Can you work these out from the drawing? Everything is in mm from the part's minimum corner. A direction names the side the tool comes from. Give positions to 0.01 mm unless a question says otherwise; leave off trailing zeros. Write each loop counter-clockwise with the first axis right and the second up, starting at its lowest first coordinate (ties: lowest second). Pieces come first, ordered by that corner, then holes. Notation, with made-up numbers: M -20,25.5 L 8,25.5 A15 ccw 8,52.5 Z; hole C 87,32 d5. An arc over 180 degrees is marked long. One line per item, written item: value.
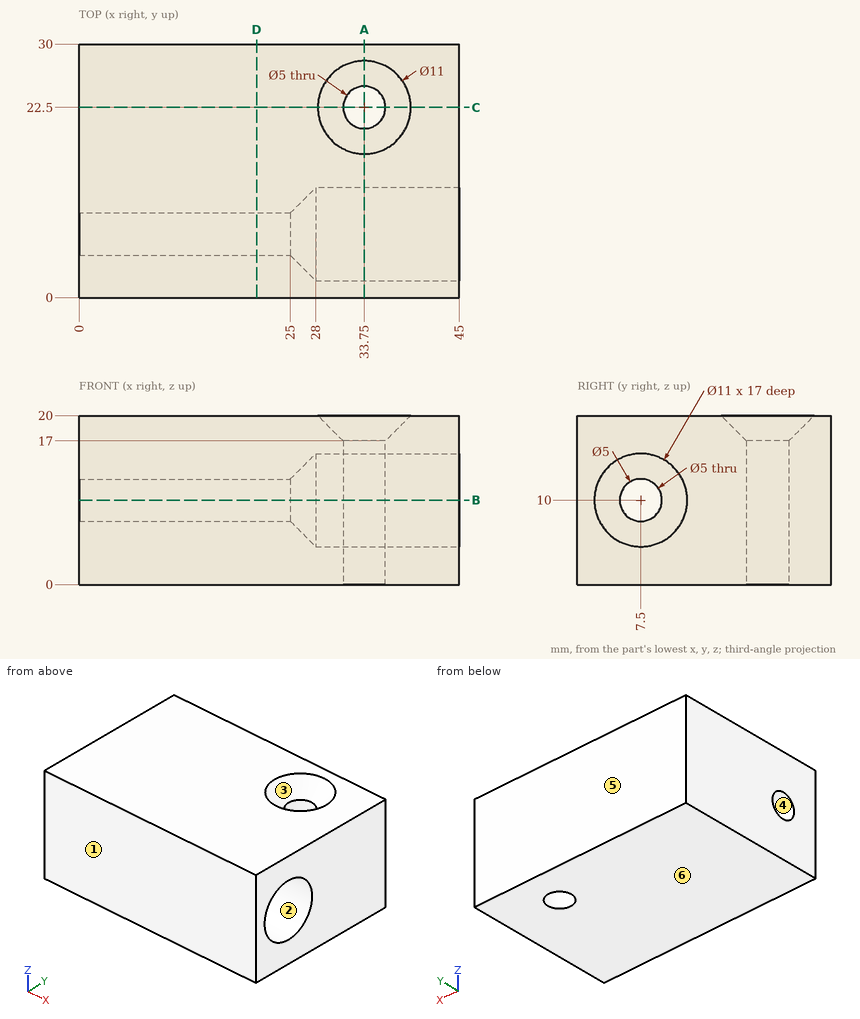
1) I'm going to push flat-ended pins straight in: pin 1 (2 mm diameter, centred on y = 7.5, z = 7.5, fed in from +X); pin 2 (9 mm diameter, centred on y = 7.5, z = 10, fed in from +X). Where does each tip first touch, or does it pass through?
Outcome:
pin 1: stops at x = 26
pin 2: stops at x = 27
2) We'd pull the mould along Y, two halves only. Please class the marked faces 3, 4, 5 and 6: pulls with the +Y half, pulls with the -Y half, needs draft (parallel to the pull), parting line crosses it, or undercut.
Outcome:
face 3: undercut
face 4: undercut
face 5: pulls with the +Y half
face 6: needs draft
3) Please list where these lines run through material, in increasing order: L1, parallel to Y at x = 33.75, z = 8.5; L2, parallel to Y at x = 33.75, z = 6.25; L3, parallel to Z at x = 8.25, y = 7.5. Write a range as from..to.
Outcome:
L1: y = 0..2.21, 12.79..20, 25..30
L2: y = 0..3.48, 11.52..20, 25..30
L3: z = 0..7.5, 12.5..20
4) If we section it at C-C, the plane y = 22.5: Write out the boundary of the cut face in (x, z).
Outcome:
outline: M 0,0 L 31.25,0 L 31.25,17 L 28.25,20 L 0,20 Z; M 36.25,0 L 45,0 L 45,20 L 39.25,20 L 36.25,17 Z
5) If we section it at D-D, the plane x = 21: Write out the boundary of the cut face in (y, z).
Outcome:
outline: M 0,0 L 30,0 L 30,20 L 0,20 Z; hole C 7.5,10 d5
6) If we section it at A-A, the plane x = 33.75: Write out the boundary of the cut face in (y, z).
Outcome:
outline: M 0,0 L 20,0 L 20,17 L 17,20 L 0,20 Z; M 25,0 L 30,0 L 30,20 L 28,20 L 25,17 Z; hole C 7.5,10 d11
7) On a 3-axis mill with a long thin cutter (end or side, diameter ignored), from which of +Z, -Z, +X, -X, +Y, -Y can I reach the whole of each face in a straight line? I mean the marked faces 1 and 2. Say none if no direction works.
Outcome:
face 1: +Z, -Z, +X, -X, -Y
face 2: +X
8) If we section it at B-B, the plane z = 10: Give the number of separate pieces and of enclosed holes in the cut face, then the cut area to 3 significant figures.
Outcome:
separate pieces: 2
enclosed holes: 1
area: 994 mm^2
